For this review, take the finished solid that the model builds, in its own axes (mm). A direction names the side the tool comes from. Coordinates: 2 decimals unless noted, no trailing zeros. Order: outer loops, then holes, each group sorted by start corner. A loop starts at its lowest first (then second) coordinate and runs counter-clockwise, first axis right, second up. Notation, with made-up numbers: M 88,33 L 100,33 A9 cw 100,48 Z; hole C 79.25,65 d3. An arc over 180 degrees is marked long. Use CSV: the item, a comma, the result in double quotes.
```python
from build123d import *

# Parameters (mm, degrees)
SKETCH_R        = 1.6
PAD_DEPTH       = 2
PAD001_DEPTH    = 22
SKETCH002_W     = 36
SKETCH002_H     = 5
PAD002_DEPTH    = 1.5
POCKET_DEPTH    = 22.001
SKETCH004_R     = 1.6
POCKET001_DEPTH = 22.001
POCKET002_DEPTH = 22.001


with BuildPart() as part:
    # Sketch → Pad (new body)
    with BuildSketch(Plane.XY):
        with BuildLine():
            Line((-32.5, 40), (56.5, 40))
            ThreePointArc((62.5, 34), (60.742641, 38.242641), (56.5, 40))
            Line((62.5, 34), (62.5, -34))
            ThreePointArc((56.5, -40), (60.742641, -38.242641), (62.5, -34))
            Line((56.5, -40), (-32.5, -40))
            ThreePointArc((-38.5, -34), (-36.742641, -38.242641), (-32.5, -40))
            Line((-38.5, -34), (-38.5, 34))
            ThreePointArc((-32.5, 40), (-36.742641, 38.242641), (-38.5, 34))
        make_face()
        with Locations((-32.5, 34)):
            Circle(SKETCH_R, mode=Mode.SUBTRACT)
        with Locations((-32.5, -34)):
            Circle(SKETCH_R, mode=Mode.SUBTRACT)
        with Locations((32.5, -34)):
            Circle(SKETCH_R, mode=Mode.SUBTRACT)
    extrude(amount=PAD_DEPTH)

    # Sketch001 → Pad001 (join)
    with BuildSketch(Plane.XY):
        Polygon((4, -4.5), (2.5, -4.5), (2.5, -21.5), (38.5, -21.5), (38.5, -26.5), (2.5, -26.5), (2.5, -28), (40, -28), (40, -20), (4, -20), align=None)
    extrude(amount=PAD001_DEPTH)

    # Sketch002 (on DatumPlane) → Pad002 (join)
    with BuildSketch(Plane.XY.offset(22)):
        with Locations((20.5, -24)):
            Rectangle(SKETCH002_W, SKETCH002_H)
    extrude(amount=-PAD002_DEPTH)

    # Sketch003 → Pocket (cut, through all)
    with BuildSketch(Plane.XY):
        with BuildLine():
            Line((-38.5, 19), (-15, 19))
            ThreePointArc((-8.5, 12.5), (-10.403806, 17.096194), (-15, 19))
            Line((-8.5, 12.5), (-8.5, -12.5))
            ThreePointArc((-15, -19), (-10.403806, -17.096194), (-8.5, -12.5))
            Line((-15, -19), (-38.5, -19))
            Line((-38.5, -19), (-38.5, 19))
        make_face()
    extrude(amount=POCKET_DEPTH, mode=Mode.SUBTRACT)

    # Sketch004 → Pocket001 (cut, through all)
    with BuildSketch(Plane.XY):
        with Locations((11, 34)):
            Circle(SKETCH004_R)
        with Locations((11, -6)):
            Circle(SKETCH004_R)
        with Locations((56, 34)):
            Circle(SKETCH004_R)
        with Locations((56, -6)):
            Circle(SKETCH004_R)
    extrude(amount=POCKET001_DEPTH, mode=Mode.SUBTRACT)

    # Sketch005 → Pocket002 (cut, through all)
    with BuildSketch(Plane.XY):
        with BuildLine():
            ThreePointArc((28.913069, 31.733732), (28.913069, 33.855052), (26.791749, 33.855052))
            Line((26.791749, 33.855052), (13.397064, 20.460367))
            ThreePointArc((13.397064, 20.460367), (13.397064, 18.339047), (15.518384, 18.339047))
            Line((28.913069, 31.733732), (15.518384, 18.339047))
        make_face()
        with BuildLine():
            ThreePointArc((39.709358, 31.178339), (39.709358, 33.29966), (37.588037, 33.29966))
            Line((37.588037, 33.29966), (11.911862, 7.623484))
            ThreePointArc((11.911862, 7.623484), (11.911862, 5.502164), (14.033182, 5.502164))
            Line((39.709358, 31.178339), (14.033182, 5.502164))
        make_face()
        with BuildLine():
            ThreePointArc((47.991417, 29.403364), (47.991417, 31.524684), (45.870097, 31.524684))
            Line((45.870097, 31.524684), (13.906073, -0.43934))
            ThreePointArc((13.906073, -0.43934), (13.906073, -2.56066), (16.027393, -2.56066))
            Line((47.991417, 29.403364), (16.027393, -2.56066))
        make_face()
        with BuildLine():
            ThreePointArc((51.769813, 21.609057), (51.769813, 23.730377), (49.648493, 23.730377))
            Line((49.648493, 23.730377), (25.136099, -0.782016))
            ThreePointArc((25.136099, -0.782016), (25.136099, -2.903337), (27.25742, -2.903337))
            Line((51.769813, 21.609057), (27.25742, -2.903337))
        make_face()
        with BuildLine():
            ThreePointArc((53.150439, 10.104192), (53.150439, 12.225512), (51.029119, 12.225512))
            Line((51.029119, 12.225512), (36.674542, -2.129064))
            ThreePointArc((36.674542, -2.129064), (36.674542, -4.250385), (38.795863, -4.250385))
            Line((53.150439, 10.104192), (38.795863, -4.250385))
        make_face()
    extrude(amount=POCKET002_DEPTH, mode=Mode.SUBTRACT)


solid = part.part
```
Item 1: To check wall thickness, follow line 1 along Y through (x, z) = (-32.5, 0.9); line 2 along X through (y, z) = (-6, 0.65); line 3 along Y through (x, z) = (11, 0.4). State the ranges of each line that lie inside material, in increasing order. Write a range as [from, to].
Solutions:
line 1,"[-40, -35.6], [-32.4, -19], [19, 32.4], [35.6, 40]"
line 2,"[-8.5, 9.4], [12.6, 54.4], [57.6, 62.5]"
line 3,"[-40, -7.6], [-4.4, 32.4], [35.6, 40]"
Item 2: For faces 1 (the face through (40, -24, 12)), 2 (the face through (20, -21.5, 11)), 3 (the face through (2.5, -14, 12)), list the 3-axis set-ups (+Z, -Z, +X, -X, +Y, -Y) from which the entire face can be reached by the end or side of a thin tool; tool diameter is ignored.
Solutions:
face 1,"+Z, +X, +Y, -Y"
face 2,"-X"
face 3,"+Z, -X, +Y, -Y"
Item 3: Draft analysis for pull direction Y (two halves, no side actions). For faces 4 (the face through (-38.5, -27, 1)), 5 (the face through (60.696, -38.289, 0.986)), 6 (the face through (37.564, 11.646, 0.986)), state which applies: released by +Y, released by -Y, zero draft, split by the parting line, or undercut.
Solutions:
face 4,"zero draft"
face 5,"released by -Y"
face 6,"undercut"
Item 4: Add section D-D on x = 5.5. State the section outline as (y, z) points, and give its area (4 significant figures).
Solutions:
outline,"M -40,0 L 40,0 L 40,2 L -20,2 L -20,22 L -28,22 L -28,2 L -40,2 Z; hole M -26.5,2 L -21.5,2 L -21.5,20.5 L -26.5,20.5 Z"
area,"227.5 mm^2"
Item 5: Add section C-C on z = 18. State the section outline as (x, y) points.
Solutions:
outline,"M 2.5,-28 L 40,-28 L 40,-20 L 4,-20 L 4,-4.5 L 2.5,-4.5 L 2.5,-21.5 L 38.5,-21.5 L 38.5,-26.5 L 2.5,-26.5 Z"
Item 6: Add section B-B on y = -6. State the section outline as (x, z) points.
Solutions:
outline,"M -8.5,0 L 9.4,0 L 9.4,2 L 4,2 L 4,22 L 2.5,22 L 2.5,2 L -8.5,2 Z; M 12.6,0 L 54.4,0 L 54.4,2 L 12.6,2 Z; M 57.6,0 L 62.5,0 L 62.5,2 L 57.6,2 Z"
Item 7: Clearance check with flat-ended pins moving along their axes: pin 1 Ø5 at (x, y) = (11, 34) entering from +Z; pin 2 Ø4 at (y, z) = (-24, 7) entering from +X; pin 3 Ø5.5 at (x, z) = (13, 7.5) entering from -Y. State where each tip first meets the part, or that it passes through.
Solutions:
pin 1,"z = 2"
pin 2,"x = 40"
pin 3,"y = -28"
Item 8: Add section A-A on x = 17.5. State the section outline as (y, z) points, and give its area (3 significant figures).
Solutions:
outline,"M -40,0 L -1.09,0 L -1.09,2 L -20,2 L -20,22 L -28,22 L -28,2 L -40,2 Z; M 3.15,0 L 8.97,0 L 8.97,2 L 3.15,2 Z; M 13.21,0 L 20.32,0 L 20.32,2 L 13.21,2 Z; M 24.56,0 L 40,0 L 40,2 L 24.56,2 Z; hole M -26.5,2 L -21.5,2 L -21.5,20.5 L -26.5,20.5 Z"
area,"202 mm^2"
